Design review of the part built by this model. Coordinates are the model's own, in mm. Face numbers are marked on the shaded views. A direction names the side the tool comes from. Round coordinates to 2 decimals unless told otherwise and drop trailing zeros. Order: outer loops, then holes, each group sorted by start corner. A loop starts at its lowest first (then second) coordinate and runs counter-clockwise, first axis right, second up.
from build123d import *

# Parameters (mm, degrees)
SKETCH1_W           = 5
SKETCH1_H           = 5
BOSS_EXTRUDE1_DEPTH = 5
CUT_EXTRUDE1_DEPTH  = 4
CUT_EXTRUDE2_DEPTH  = 1
SKETCH5_W           = 2
SKETCH5_H           = 2
CUT_EXTRUDE9_DEPTH  = 3
CUT_EXTRUDE10_DEPTH = 2
SKETCH11_W          = 1
SKETCH11_H          = 2
CUT_EXTRUDE11_DEPTH = 2
CUT_EXTRUDE14_DEPTH = 5
CUT_EXTRUDE15_DEPTH = 2
CUT_EXTRUDE16_DEPTH = 2


with BuildPart() as part:
    # Sketch1 → Boss-Extrude1 (new body)
    with BuildSketch(Plane.XY):
        Rectangle(SKETCH1_W, SKETCH1_H)
    extrude(amount=BOSS_EXTRUDE1_DEPTH)

    # Sketch2 → Cut-Extrude1 (cut)
    with BuildSketch(Plane(origin=(0, 2.5, 0), x_dir=(1, 0, 0), z_dir=(0, 1, 0))):
        Polygon((2.5, -5), (2.5, -3), (0.5, -5), align=None)
    extrude(amount=-CUT_EXTRUDE1_DEPTH, mode=Mode.SUBTRACT)

    # Sketch4 → Cut-Extrude2 (cut)
    with BuildSketch(Plane.ZY.offset(2.5)):
        Polygon((5, 2.5), (4, 2.5), (5, 0.5), align=None)
    extrude(amount=-CUT_EXTRUDE2_DEPTH, mode=Mode.SUBTRACT)

    # Sketch5 → Cut-Extrude9 (cut)
    with BuildSketch(Plane.XY.offset(5)):
        with Locations((1.5, 1.5)):
            Rectangle(SKETCH5_W, SKETCH5_H)
    extrude(amount=-CUT_EXTRUDE9_DEPTH, mode=Mode.SUBTRACT)

    # Sketch10 → Cut-Extrude10 (cut)
    with BuildSketch(Plane(origin=(2.5, 0, 0), x_dir=(0, 0, -1), z_dir=(1, 0, 0))):
        Polygon((-1, 2.5), (-2, 0.5), (-2, 2.5), align=None)
    extrude(amount=-CUT_EXTRUDE10_DEPTH, mode=Mode.SUBTRACT)

    # Sketch11 → Cut-Extrude11 (cut)
    with BuildSketch(Plane(origin=(0.5, 0, 0), x_dir=(0, 0, -1), z_dir=(1, 0, 0))):
        with Locations((-4.5, 1.5)):
            Rectangle(SKETCH11_W, SKETCH11_H)
    extrude(amount=-CUT_EXTRUDE11_DEPTH, mode=Mode.SUBTRACT)

    # Sketch16 → Cut-Extrude14 (cut, through all)
    with BuildSketch(Plane(origin=(1.222222222, 0.611111111, 1.222222222), x_dir=(-0.745355992, 0.298142397, 0.596284794), z_dir=(-0.666666667, -0.333333333, -0.666666667))):
        Polygon((0.96896279, -0.447213595), (0.96896279, 1.788854382), (3.652244363, 0.894427191), (3.652244363, -1.341640786), align=None)
    extrude(amount=-CUT_EXTRUDE14_DEPTH, mode=Mode.SUBTRACT)

    # Sketch17 → Cut-Extrude15 (cut)
    with BuildSketch(Plane(origin=(-1.5, 0, 0), x_dir=(0, 0, -1), z_dir=(1, 0, 0))):
        Polygon((-3, 2.5), (-4, 0.5), (-4, 2.5), align=None)
    extrude(amount=CUT_EXTRUDE15_DEPTH, mode=Mode.SUBTRACT)

    # Sketch18 → Cut-Extrude16 (cut)
    with BuildSketch(Plane(origin=(0, 0.5, 0), x_dir=(1, 0, 0), z_dir=(0, 1, 0))):
        Polygon((0.5, -4), (0.5, -2), (-1.5, -4), align=None)
    extrude(amount=CUT_EXTRUDE16_DEPTH, mode=Mode.SUBTRACT)


solid = part.part
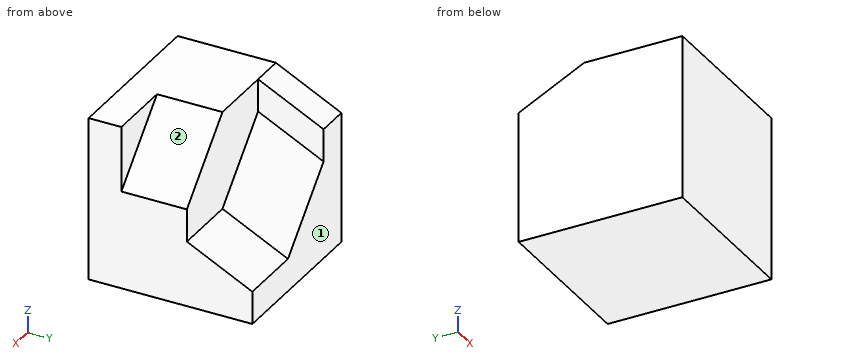
1) Clearance check with a flat-ended pin moving along its axis: P1, Ø1, axis at x = 1.5, z = 4, coming from the +Y side. State where the tip first meets the part, or that it passes through.
Results:
P1: stops at y = 0.5
2) Take a section at A-A on x = 1.35. Give the boundary of the cut face in (y, z), plus the area to 3 significant figures.
Results:
outline: (-2.5, 0) - (2.5, 0) - (2.5, 1) - (0.5, 2) - (0.5, 4.15) - (-1.5, 4.15) - (-1.5, 5) - (-2.5, 5) - close
area: 16.3 mm2
3) Take a section at D-D on x = 0.65. Give the boundary of the cut face in (y, z), plus the area to 3 significant figures.
Results:
outline: (-2.5, 0) - (2.5, 0) - (2.5, 1) - (0.5, 2) - (0.5, 4.85) - (-1.5, 4.85) - (-1.5, 5) - (-2.5, 5) - close
area: 17.7 mm2
4) For the marked faces 1 and 2, list the 3-axis set-ups (+Z, -Z, +X, -X, +Y, -Y) from which the entire face can be reached by the end or side of a thin tool; tool diameter is ignored.
Results:
face 1: +Z, -Z, +X, -X, +Y
face 2: +Z, +X, +Y
5) To check wall thickness, follow line 1 along X through (y, z) = (1.75, 4.2); line 2 along Y through (x, z) = (1.05, 3.4). State the ranges of each line that lie inside material, in increasing order.
Results:
line 1: x = -2.5 to -1.5
line 2: y = -2.5 to 0.5
6) Take a section at B-B on z = 1.9. Give the boundary of the cut face in (x, y).
Results:
outline: (-2.5, -2.5) - (2.5, -2.5) - (2.5, 0.7) - (0.5, 0.7) - (-0.4, 2.5) - (-2.5, 2.5) - close
7) Take a section at C-C on y = 1.65. Give the boundary of the cut face in (x, z) (3 decimals).
Results:
outline: (-2.5, 0) - (2.5, 0) - (2.5, 1.425) - (0.5, 1.425) - (-1.5, 3.425) - (-1.5, 4.425) - (-2.5, 4.425) - close
